```python
from build123d import *

# Parameters (mm, degrees)
CROQUIS1_W                         = 431.038
CROQUIS1_H                         = 254
BRIDA_BASE1_DEPTH                  = 1.524
CORTAR_EXTRUIR1_REACH              = 252.159
CROQUIS6_W                         = 4.826
CROQUIS6_H                         = 4.826
BRIDA_DE_ARISTA1_STRIP_W           = 9.144
BRIDA_DE_ARISTA1_STRIP_H           = 1.524
BRIDA_DE_ARISTA1_STRIP_CUT_DEPTH   = 426.212
BRIDA_DE_ARISTA1_STRIP_2_W         = 9.144
BRIDA_DE_ARISTA1_STRIP_2_H         = 1.524
BRIDA_DE_ARISTA1_STRIP_CUT_2_DEPTH = 426.212
BRIDA_DE_ARISTA1_STRIP_3_W         = 9.144
BRIDA_DE_ARISTA1_STRIP_3_H         = 1.524
BRIDA_DE_ARISTA1_STRIP_CUT_3_DEPTH = 244.348
BRIDA_DE_ARISTA1_DEPTH             = 426.212
BRIDA_DE_ARISTA1_BEND_DEPTH        = 426.212
BRIDA_DE_ARISTA1_BEND_2_DEPTH      = 244.348
CORTAR_EXTRUIR2_REACH              = 252.666
CROQUIS16_R                        = 3.9624
CROQUIS16_R_2                      = 2.8956
CROQUIS16_R_3                      = 2.413


# Sheet-metal steps are written as plain solids
with BuildPart() as part:
    # Croquis1 → Brida base1 (new body)
    with BuildSketch(Plane.XY):
        Rectangle(CROQUIS1_W, CROQUIS1_H)
    extrude(amount=-BRIDA_BASE1_DEPTH)

    # Croquis6 → Cortar-Extruir1 (cut, up to next)
    with BuildSketch(Plane.XY, mode=Mode.PRIVATE) as cortar_extruir1_sk1:
        with Locations((-213.106, 124.587)):
            Rectangle(CROQUIS6_W, CROQUIS6_H)
    cortar_extruir1_tool1 = extrude(cortar_extruir1_sk1.sketch, amount=-CORTAR_EXTRUIR1_REACH, mode=Mode.PRIVATE) & part.part
    # Croquis6 → Cortar-Extruir1 (cut, up to next)
    with BuildSketch(Plane.XY, mode=Mode.PRIVATE) as cortar_extruir1_sk2:
        with Locations((-213.106, -124.587)):
            Rectangle(CROQUIS6_W, CROQUIS6_H)
    cortar_extruir1_tool2 = extrude(cortar_extruir1_sk2.sketch, amount=-CORTAR_EXTRUIR1_REACH, mode=Mode.PRIVATE) & part.part
    add(cortar_extruir1_tool1.solids().sort_by_distance((-213.106, 124.587, 0))[0], mode=Mode.SUBTRACT)
    add(cortar_extruir1_tool2.solids().sort_by_distance((-213.106, -124.587, 0))[0], mode=Mode.SUBTRACT)

    # Brida de arista1 strip (across the edge) → Brida de arista1 strip cut (cut)
    with BuildSketch(Plane(origin=(-210.693, 127, -1.524), x_dir=(0, -1, 0), z_dir=(1, 0, 0))):
        with Locations((-1.524, -0.762)):
            Rectangle(BRIDA_DE_ARISTA1_STRIP_W, BRIDA_DE_ARISTA1_STRIP_H)
    extrude(amount=BRIDA_DE_ARISTA1_STRIP_CUT_DEPTH, mode=Mode.SUBTRACT)

    # Brida de arista1 strip 2 (across the edge) → Brida de arista1 strip cut 2 (cut)
    with BuildSketch(Plane(origin=(215.519, -127, -1.524), x_dir=(0, 1, 0), z_dir=(-1, 0, 0))):
        with Locations((-1.524, -0.762)):
            Rectangle(BRIDA_DE_ARISTA1_STRIP_2_W, BRIDA_DE_ARISTA1_STRIP_2_H)
    extrude(amount=BRIDA_DE_ARISTA1_STRIP_CUT_2_DEPTH, mode=Mode.SUBTRACT)

    # Brida de arista1 strip 3 (across the edge) → Brida de arista1 strip cut 3 (cut)
    with BuildSketch(Plane(origin=(-215.519, -122.174, -1.524), x_dir=(1, 0, 0), z_dir=(0, 1, 0))):
        with Locations((-1.524, -0.762)):
            Rectangle(BRIDA_DE_ARISTA1_STRIP_3_W, BRIDA_DE_ARISTA1_STRIP_3_H)
    extrude(amount=BRIDA_DE_ARISTA1_STRIP_CUT_3_DEPTH, mode=Mode.SUBTRACT)

    # Brida de arista1 section (across the edge) → Brida de arista1 (add)
    with BuildSketch(Plane(origin=(-210.693, 127, -1.524), x_dir=(0, -1, 0), z_dir=(1, 0, 0))):
        with BuildLine():
            Line((0, 1.524), (0, 14.478))
            Line((0, 14.478), (1.524, 14.478))
            Line((1.524, 14.478), (1.524, 1.524))
            ThreePointArc((1.524, 1.524), (1.970369265, 0.446369265), (3.048, 0))
            Line((3.048, 0), (3.048, -1.524))
            ThreePointArc((3.048, -1.524), (0.892738531, -0.631261469), (0, 1.524))
        make_face()
    extrude(amount=BRIDA_DE_ARISTA1_DEPTH)

    # Brida de arista1 section 2 (across the edge) → Brida de arista1 bend (add)
    with BuildSketch(Plane(origin=(215.519, -127, -1.524), x_dir=(0, 1, 0), z_dir=(-1, 0, 0))):
        with BuildLine():
            Line((0, 1.524), (0, 14.478))
            Line((0, 14.478), (1.524, 14.478))
            Line((1.524, 14.478), (1.524, 1.524))
            ThreePointArc((1.524, 1.524), (1.970369265, 0.446369265), (3.048, 0))
            Line((3.048, 0), (3.048, -1.524))
            ThreePointArc((3.048, -1.524), (0.892738531, -0.631261469), (0, 1.524))
        make_face()
    extrude(amount=BRIDA_DE_ARISTA1_BEND_DEPTH)

    # Brida de arista1 section 3 (across the edge) → Brida de arista1 bend 2 (add)
    with BuildSketch(Plane(origin=(-215.519, -122.174, -1.524), x_dir=(1, 0, 0), z_dir=(0, 1, 0))):
        with BuildLine():
            Line((0, 1.524), (0, 14.478))
            Line((0, 14.478), (1.524, 14.478))
            Line((1.524, 14.478), (1.524, 1.524))
            ThreePointArc((1.524, 1.524), (1.970369265, 0.446369265), (3.048, 0))
            Line((3.048, 0), (3.048, -1.524))
            ThreePointArc((3.048, -1.524), (0.892738531, -0.631261469), (0, 1.524))
        make_face()
    extrude(amount=BRIDA_DE_ARISTA1_BEND_2_DEPTH)

    # Croquis16 → Cortar-Extruir2 (cut, up to next)
    with BuildSketch(Plane.XY, mode=Mode.PRIVATE) as cortar_extruir2_sk1:
        with Locations((-202.819, 0)):
            Circle(CROQUIS16_R)
    cortar_extruir2_tool1 = extrude(cortar_extruir2_sk1.sketch, amount=-CORTAR_EXTRUIR2_REACH, mode=Mode.PRIVATE) & part.part
    # Croquis16 → Cortar-Extruir2 (cut, up to next)
    with BuildSketch(Plane.XY, mode=Mode.PRIVATE) as cortar_extruir2_sk2:
        with Locations((-167.767, 60.452)):
            Circle(CROQUIS16_R_2)
    cortar_extruir2_tool2 = extrude(cortar_extruir2_sk2.sketch, amount=-CORTAR_EXTRUIR2_REACH, mode=Mode.PRIVATE) & part.part
    # Croquis16 → Cortar-Extruir2 (cut, up to next)
    with BuildSketch(Plane.XY, mode=Mode.PRIVATE) as cortar_extruir2_sk3:
        with Locations((-167.767, -60.452)):
            Circle(CROQUIS16_R_2)
    cortar_extruir2_tool3 = extrude(cortar_extruir2_sk3.sketch, amount=-CORTAR_EXTRUIR2_REACH, mode=Mode.PRIVATE) & part.part
    # Croquis16 → Cortar-Extruir2 (cut, up to next)
    with BuildSketch(Plane.XY, mode=Mode.PRIVATE) as cortar_extruir2_sk4:
        with Locations((207.645, 88.9)):
            Circle(CROQUIS16_R_3)
    cortar_extruir2_tool4 = extrude(cortar_extruir2_sk4.sketch, amount=-CORTAR_EXTRUIR2_REACH, mode=Mode.PRIVATE) & part.part
    # Croquis16 → Cortar-Extruir2 (cut, up to next)
    with BuildSketch(Plane.XY, mode=Mode.PRIVATE) as cortar_extruir2_sk5:
        with Locations((207.645, 0)):
            Circle(CROQUIS16_R_3)
    cortar_extruir2_tool5 = extrude(cortar_extruir2_sk5.sketch, amount=-CORTAR_EXTRUIR2_REACH, mode=Mode.PRIVATE) & part.part
    # Croquis16 → Cortar-Extruir2 (cut, up to next)
    with BuildSketch(Plane.XY, mode=Mode.PRIVATE) as cortar_extruir2_sk6:
        with Locations((207.645, -88.9)):
            Circle(CROQUIS16_R_3)
    cortar_extruir2_tool6 = extrude(cortar_extruir2_sk6.sketch, amount=-CORTAR_EXTRUIR2_REACH, mode=Mode.PRIVATE) & part.part
    add(cortar_extruir2_tool1.solids().sort_by_distance((-202.819, 0, 0))[0], mode=Mode.SUBTRACT)
    add(cortar_extruir2_tool2.solids().sort_by_distance((-167.767, 60.452, 0))[0], mode=Mode.SUBTRACT)
    add(cortar_extruir2_tool3.solids().sort_by_distance((-167.767, -60.452, 0))[0], mode=Mode.SUBTRACT)
    add(cortar_extruir2_tool4.solids().sort_by_distance((207.645, 88.9, 0))[0], mode=Mode.SUBTRACT)
    add(cortar_extruir2_tool5.solids().sort_by_distance((207.645, 0, 0))[0], mode=Mode.SUBTRACT)
    add(cortar_extruir2_tool6.solids().sort_by_distance((207.645, -88.9, 0))[0], mode=Mode.SUBTRACT)


solid = part.part
```
Source: CAD feature listing. Evaluate the final solid. Frame: model axes, mm. A direction names the side the tool comes from. Give positions to 0.01 mm unless a question says otherwise; leave off trailing zeros. Order: outer loops, then holes, each group sorted by start corner. A loop starts at its lowest first (then second) coordinate and runs counter-clockwise, first axis right, second up.
(1) Section query A-A (z = -6.25). Return the cut outline in (x, y) (3 decimals).
(2) Section query B-B (y = -102.5). Return the cut outline in (x, z) (3 decimals).
(3) Contact query for flat-ended pins moving along their axis: P1, Ø4.5, axis at x = 207.645, y = 0, coming from the -Z side; P2, Ø1.4, axis at y = 125.5, z = -8.5, coming from the -X side; P3, Ø2, axis at y = -99, z = -2, coming from the +X side; P4, Ø2.5, axis at x = -213, z = -9, coming from the +Y side. Output: stop coordinate, or through.
(4) Material intervals for line 1 along Y through (x, z) = (-101, -12.75); line 2 along Z through (x, y) = (-108, -37); line 3 along X through (y, z) = (64, -8) (3 decimals), sorted ascending.
(5) Section query C-C (x = 133). Return the cut outline in (y, z).
(6) Pull-direction query (X, two-part tool) for faces 4 (the face through (-215.519, -2, -9)), 5 (the face through (-1, 125.476, -10)), 6 (the face through (-199.04, 1.19, -0.75)); classes: +X half, -X half, draft (parallel to the pull), parting line (faces both ways), or undercut.
(7) Access query for faces 1 (the face through (-1, 2, -1.524)), 2 (the face through (-213.995, -2, -10)), 3 (the face through (5, -125.476, -10)). Directions: +Z, -Z, +X, -X, +Y, -Y. A direction counts if a zero-diameter tool reaches every point of the face in a straight line with its end or side. Return the directions, or none.
Outcome:
1. outline: (-215.519, -122.174) - (-213.995, -122.174) - (-213.995, 122.174) - (-215.519, 122.174) - close; (-210.693, -127) - (215.519, -127) - (215.519, -125.476) - (-210.693, -125.476) - close; (-210.693, 125.476) - (215.519, 125.476) - (215.519, 127) - (-210.693, 127) - close
2. outline: (-215.519, -16.002) - (-213.995, -16.002) - (-213.995, -3.048) arc R1.524 cw to (-212.471, -1.524) - (215.519, -1.524) - (215.519, 0) - (-212.471, 0) arc R3.048 ccw to (-215.519, -3.048) - close
3. P1: passes through
3. P2: stops at x = -210.69
3. P3: stops at x = 215.52
3. P4: stops at y = 122.17
4. line 1: y = -127 to -125.48, 125.48 to 127
4. line 2: z = -1.52 to 0
4. line 3: x = -215.519 to -213.995
5. outline: (-127, -16) - (-125.48, -16) - (-125.48, -3.05) arc R1.52 cw to (-123.95, -1.52) - (123.95, -1.52) arc R1.52 cw to (125.48, -3.05) - (125.48, -16) - (127, -16) - (127, -3.05) arc R3.05 ccw to (123.95, 0) - (-123.95, 0) arc R3.05 ccw to (-127, -3.05) - close
6. face 4: -X half
6. face 5: draft
6. face 6: undercut
7. face 1: -Z, +X
7. face 2: -Z, +X, +Y, -Y
7. face 3: -Z, +X, -X
